Geometry: see drawing. Coordinates: mm, zero at the bounding-box minimum. A direction names the side the tool comes from. Round coordinates to 2 decimals unless told otherwise and drop trailing zeros. Write each loop counter-clockwise with the first axis right and the second up, starting at its lowest first coordinate (ties: lowest second). Pieces come first, ordered by that corner, then holes. Notation, with made-up numbers: (82.25, 20.5) -> (103.25, 20.5) arc R31 ccw to (103.25, 46.5) -> close; hole circle Ø3 at (60, 66). An arc over 180 degrees is marked (long way). Use CSV: the item, a comma, the result in double quotes.
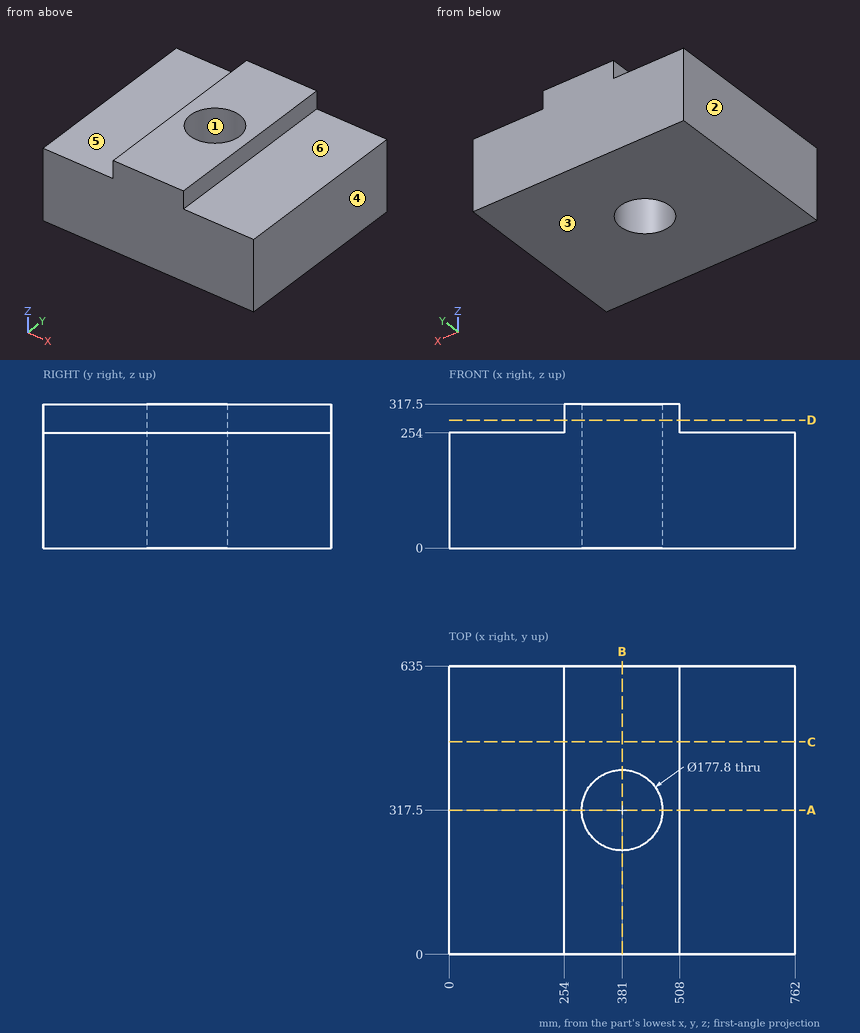
Item 1: Pull-direction query (X, two-part tool) for the marked faces 1, 2 and 3; classes: +X half, -X half, draft (parallel to the pull), parting line (faces both ways), or undercut.
Worked answers:
face 1,"undercut"
face 2,"-X half"
face 3,"draft"
Item 2: Section query A-A on y = 317.5. Return the cut outline in (x, z), plus the area to 3 significant figures.
Worked answers:
outline,"(0, 0) -> (292.1, 0) -> (292.1, 317.5) -> (254, 317.5) -> (254, 254) -> (0, 254) -> close; (469.9, 0) -> (762, 0) -> (762, 254) -> (508, 254) -> (508, 317.5) -> (469.9, 317.5) -> close"
area,"153,000 mm²"
Item 3: Line query: line 1 (X direction, y = 317, z = 70); line 2 (Y direction, x = 381, z = 228); line 3 (X direction, y = 340.5, z = 70). Output: solid intervals per line, ascending.
Worked answers:
line 1,"x = 0 to 292.1, 469.9 to 762"
line 2,"y = 0 to 228.6, 406.4 to 635"
line 3,"x = 0 to 295.13, 466.87 to 762"
Item 4: First-contact query: pin 1 Ø1 at (x, y) = (659, 204.5) entering from +Z. Flat tip, straight axial feed; report the tip coordinate or a pass-through.
Worked answers:
pin 1,"stops at z = 254"
Item 5: Set-up query: the marked faces 4, 5 and 6. Return all of +Z, -Z, +X, -X, +Y, -Y with unobstructed straight access to the full face (end or side cutting, diameter ignored); none if empty.
Worked answers:
face 4,"+Z, -Z, +X, +Y, -Y"
face 5,"+Z, -X, +Y, -Y"
face 6,"+Z, +X, +Y, -Y"
Item 6: Section query D-D on z = 282. Return the cut outline in (x, y).
Worked answers:
outline,"(254, 0) -> (508, 0) -> (508, 635) -> (254, 635) -> close; hole circle Ø177.8 at (381, 317.5)"
Item 7: Section query B-B on x = 381. Return the cut outline in (y, z), plus the area to 3 significant figures.
Worked answers:
outline,"(0, 0) -> (228.6, 0) -> (228.6, 317.5) -> (0, 317.5) -> close; (406.4, 0) -> (635, 0) -> (635, 317.5) -> (406.4, 317.5) -> close"
area,"145,000 mm²"
Item 8: Section query C-C on y = 468. Return the cut outline in (x, z).
Worked answers:
outline,"(0, 0) -> (762, 0) -> (762, 254) -> (508, 254) -> (508, 317.5) -> (254, 317.5) -> (254, 254) -> (0, 254) -> close"
